The model under review builds one solid part; all positions refer to its coordinate system, in mm. A direction names the side the tool comes from. Coordinates: 2 decimals unless noted, no trailing zeros. Write each loop counter-clockwise with the first axis right and the second up, starting at its lowest first coordinate (ties: lowest second). Pieces come first, ordered by that corner, then holes. Notation, with made-up numbers: M 47,89.5 L 106,89.5 A26 cw 106,115.5 Z; hole C -34.5,44.5 d5. An arc over 180 degrees is marked long. Answer as a JSON object with one key per item and string values.
```python
from build123d import *

# Parameters (mm, degrees)
SKETCH1_W                      = 89.535
SKETCH1_H                      = 76.2
EXTRUDE1_DEPTH                 = 9.525
CBORE_FOR_M5_SHCS3_D           = 5.5
CBORE_FOR_M5_SHCS3_CBORE_D     = 10
CBORE_FOR_M5_SHCS3_CBORE_DEPTH = 5
LPATTERN4_COUNT                = 2
LPATTERN4_PITCH                = 63.5
LPATTERN4_COUNT_DIR2           = 2
LPATTERN4_PITCH_DIR2           = 25.4
M3X0_5_TAPPED_HOLE2_D          = 2.5
LPATTERN5_COUNT                = 2
LPATTERN5_PITCH                = 83.185
LPATTERN5_COUNT_DIR2           = 2
LPATTERN5_PITCH_DIR2           = 69.85


with BuildPart() as part:
    # Sketch1 → Extrude1 (new body)
    with BuildSketch(Plane(origin=(0, 0, 0), x_dir=(1, 0, 0), z_dir=(0, 1, 0))):
        Rectangle(SKETCH1_W, SKETCH1_H)
    extrude(amount=EXTRUDE1_DEPTH)

    # CBORE for M5 SHCS3 (through all)
    with Locations(Plane(origin=(-31.75, 9.525, 31.75), x_dir=(0, 0, 1), z_dir=(0, 1, 0))):
        with Locations((0, 0)):
            cbore_for_m5_shcs3 = CounterBoreHole(CBORE_FOR_M5_SHCS3_D / 2, CBORE_FOR_M5_SHCS3_CBORE_D / 2, CBORE_FOR_M5_SHCS3_CBORE_DEPTH)

    # LPattern4: CBORE for M5 SHCS3 2 × 2
    with Locations(*[(i * LPATTERN4_PITCH, 0, -j * LPATTERN4_PITCH_DIR2) for i in range(LPATTERN4_COUNT) for j in range(LPATTERN4_COUNT_DIR2) if (i, j) != (0, 0)]):
        add(cbore_for_m5_shcs3, mode=Mode.SUBTRACT)

    # M3x0.5 Tapped Hole2 (through all)
    with Locations(Plane(origin=(-41.5925, 9.525, 34.925), x_dir=(0, 0, 1), z_dir=(0, 1, 0))):
        with Locations((0, 0)):
            m3x0_5_tapped_hole2 = Hole(M3X0_5_TAPPED_HOLE2_D / 2)

    # LPattern5: M3x0.5 Tapped Hole2 2 × 2
    with Locations(*[(i * LPATTERN5_PITCH, 0, -j * LPATTERN5_PITCH_DIR2) for i in range(LPATTERN5_COUNT) for j in range(LPATTERN5_COUNT_DIR2) if (i, j) != (0, 0)]):
        add(m3x0_5_tapped_hole2, mode=Mode.SUBTRACT)


solid = part.part
```
(1) For pin 1 Ø3 at (x, z) = (31.5, 8) entering from +Y (3 decimals), flat-tipped, find the tip position at first contact; note if it passes through.
Results list:
{"pin 1": "y = 4.525"}
(2) Add section A-A on x = -31.75. Give the boundary of the cut face in (y, z) (3 decimals), and give its area (3 significant figures).
Results list:
{"outline": "M 0,-38.1 L 9.525,-38.1 L 9.525,1.35 L 4.525,1.35 L 4.525,3.6 L 0,3.6 Z; M 0,9.1 L 4.525,9.1 L 4.525,11.35 L 9.525,11.35 L 9.525,26.75 L 4.525,26.75 L 4.525,29 L 0,29 Z; M 0,34.5 L 4.525,34.5 L 4.525,36.75 L 9.525,36.75 L 9.525,38.1 L 0,38.1 Z", "area": "576 mm²"}
(3) For faces 5 (the face through (-36.63, 7.06, 5.27)), 6 (the face through (33.609, 2.231, 33.777)), list the 3-axis set-ups (+Z, -Z, +X, -X, +Y, -Y) from which the entire face can be reached by the end or side of a thin tool; tool diameter is ignored.
Results list:
{"face 5": "+Y", "face 6": "+Y, -Y"}
(4) Wall thickness on line 1 along X through (y, z) = (1.5, 6); line 2 along X through (y, z) = (7.5, 32.5): over which ranges is each line inside the solid? List them lowest first. Write a range as from..to.
Results list:
{"line 1": "-44.77..-34.48, -29.02..29.02, 34.48..44.77", "line 2": "-44.77..-36.69, -26.81..26.81, 36.69..44.77"}
(5) Draft analysis for pull direction Z (two halves, no side actions). For faces 1 (the face through (42.83, 4.7, 35.09)), 2 (the face through (-1, 5, 38.1)), 3 (the face through (-34, 4.525, 34)), 4 (the face through (44.768, 5, 1)), state which applies: released by +Z, released by -Z, zero draft, split by the parting line, or undercut.
Results list:
{"face 1": "undercut", "face 2": "released by +Z", "face 3": "undercut", "face 4": "zero draft"}
(6) Add section B-B on z = 31.75. Count the separate pieces of the cut face and the enclosed holes in it, and give its area (3 significant figures).
Results list:
{"separate pieces": "3", "enclosed holes": "0", "area": "703 mm²"}
